Check sheet for the drawn part. Datum: minimum x, y, z corner. Units: mm. A direction names the side the tool comes from. Round coordinates to 2 decimals unless told otherwise and drop trailing zeros. Order: outer loops, then holes, each group sorted by start corner. A loop starts at its lowest first (then second) coordinate and runs counter-clockwise, first axis right, second up. Notation, with made-up numbers: (10, 29) -> (40, 29) arc R24 cw to (40, 48) -> close; hole circle Ø11 at (54, 42). An arc over 180 degrees is marked (long way). Use CSV: the item, a comma, the result in double quotes.
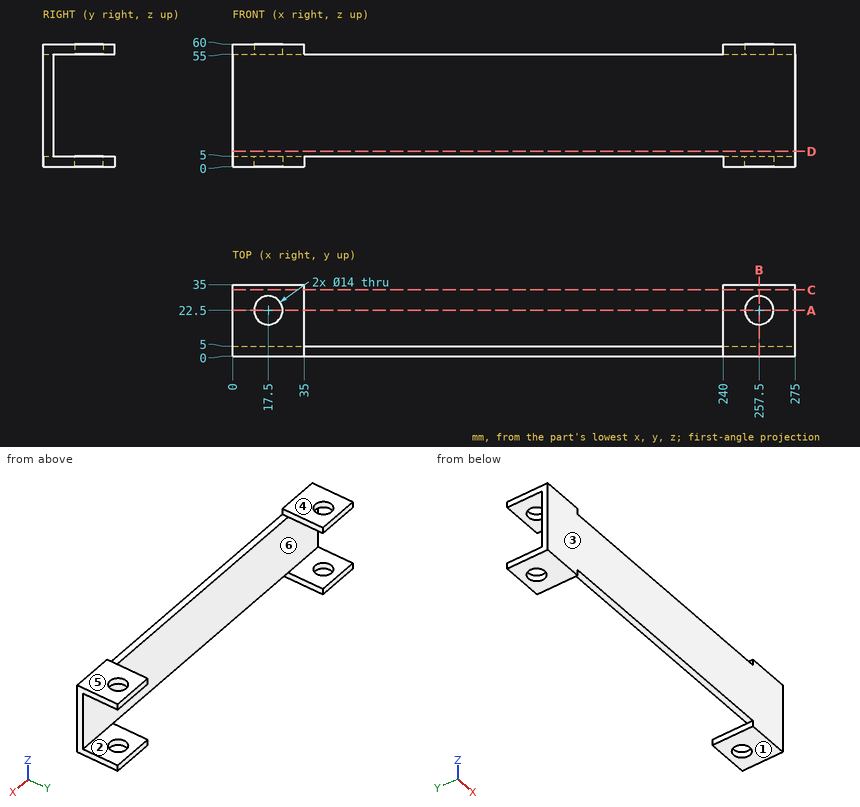
Q1. Mould release check, pull along Z, two halves, no side actions. Record for the marked faces 1, 2, 3 and 4: pulls with the +Z half, pulls with the -Z half, needs draft (parallel to the pull), parting line crosses it, or undercut.
Result sheet:
face 1,"pulls with the -Z half"
face 2,"undercut"
face 3,"needs draft"
face 4,"pulls with the +Z half"
Q2. Sectioned sample at D-D, the plane z = 7.5. Enter the section's corners in (x, y), then the cut area to 4 significant figures.
Result sheet:
outline,"(0, 0) -> (275, 0) -> (275, 5) -> (0, 5) -> close"
area,"1,375 mm^2"
Q3. Go/stop test with flat-tipped pins: pin 1 (2.5 mm diameter, centred on x = 92.5, y = 2.5, fed in from +Z); pin 2 (1.5 mm diameter, centred on x = 156.5, y = 1.5, fed in from -Z); pin 3 (25 mm diameter, centred on x = 185, z = 31, fed in from +Y). Record where each tip stops, or that it passes through.
Result sheet:
pin 1,"stops at z = 55"
pin 2,"stops at z = 5"
pin 3,"stops at y = 5"
Q4. Sectioned sample at A-A, the plane y = 22.5. State how many separate pieces and enclosed holes the cut face has, then the cut area to 3 significant figures.
Result sheet:
separate pieces,"8"
enclosed holes,"0"
area,"420 mm^2"
Q5. Scan lines: L1, parallel to X at y = 22, z = 57; L2, parallel to Y at x = 257, z = 57; L3, parallel to X at y = 20, z = 3. Record each from-to range of solid material in increasing order.
Result sheet:
L1,"x = 0 to 10.52, 24.48 to 35, 240 to 250.52, 264.48 to 275"
L2,"y = 0 to 15.52, 29.48 to 35"
L3,"x = 0 to 10.96, 24.04 to 35, 240 to 250.96, 264.04 to 275"
Q6. Sectioned sample at C-C, the plane y = 32.5. Enter the section's corners in (x, z), then the cut area to 3 significant figures.
Result sheet:
outline,"(0, 0) -> (35, 0) -> (35, 5) -> (0, 5) -> close; (0, 55) -> (35, 55) -> (35, 60) -> (0, 60) -> close; (240, 0) -> (275, 0) -> (275, 5) -> (240, 5) -> close; (240, 55) -> (275, 55) -> (275, 60) -> (240, 60) -> close"
area,"700 mm^2"
Q7. Sectioned sample at B-B, the plane x = 257.5. Enter the section's corners in (y, z).
Result sheet:
outline,"(0, 0) -> (15.5, 0) -> (15.5, 5) -> (5, 5) -> (5, 55) -> (15.5, 55) -> (15.5, 60) -> (0, 60) -> close; (29.5, 0) -> (35, 0) -> (35, 5) -> (29.5, 5) -> close; (29.5, 55) -> (35, 55) -> (35, 60) -> (29.5, 60) -> close"
Q8. Access from +Z, -Z, +X, -X, +Y, -Y to the whole of each face (thin tool, end or side, straight path). Record for the marked faces 5 and 6.
Result sheet:
face 5,"+Z, +X, -X, +Y, -Y"
face 6,"+X, -X, +Y"
